from build123d import *

# Parameters (mm, degrees)
F0_R     = 29.980607
F1_DEPTH = 31.75
F2_DEPTH = 17.78
F4_DEPTH = 5.08


with BuildPart() as f1:
    # F0 (on Top) → F1 (new body)
    with BuildSketch(Plane.XY):
        with BuildLine():
            ThreePointArc((8.249651, -24.887905), (54.774032, -39.548346), (83.328802, 0))
            ThreePointArc((83.328802, 0), (54.774032, 39.548346), (8.249651, 24.887905))
            ThreePointArc((8.249651, 24.887905), (2.145128, 13.197838), (0, 0.185486))
            Line((0, 0.185486), (0, 0))
            Line((0, 0), (0, -0.185486))
            ThreePointArc((0, -0.185486), (2.145128, -13.197838), (8.249651, -24.887905))
        make_face()
        with Locations((41.664194, 0)):
            Circle(F0_R, mode=Mode.SUBTRACT)
    extrude(amount=F1_DEPTH)

    # F0 (on Top) → F2 (join)
    with BuildSketch(Plane.XY):
        with BuildLine():
            ThreePointArc((8.249651, -24.887905), (54.774032, -39.548346), (83.328802, 0))
            ThreePointArc((83.328802, 0), (54.774032, 39.548346), (8.249651, 24.887905))
            ThreePointArc((8.249651, 24.887905), (2.145128, 13.197838), (0, 0.185486))
            Line((0, 0.185486), (0, 0))
            Line((0, 0), (0, -0.185486))
            ThreePointArc((0, -0.185486), (2.145128, -13.197838), (8.249651, -24.887905))
        make_face()
        with Locations((41.664194, 0)):
            Circle(F0_R, mode=Mode.SUBTRACT)
        with BuildLine():
            ThreePointArc((0, 0.185486), (2.145128, 13.197838), (8.249651, 24.887905))
            Line((8.249651, 24.887905), (0, 24.887905))
            Line((0, 24.887905), (0, 0.185486))
        make_face()
        with BuildLine():
            Line((0, -24.887905), (8.249651, -24.887905))
            ThreePointArc((8.249651, -24.887905), (2.145128, -13.197838), (0, -0.185486))
            Line((0, -0.185486), (0, -24.887905))
        make_face()
        with BuildLine():
            ThreePointArc((-0.000413, 0), (-0.00031, 0.092743), (0, 0.185486))
            Line((0, 0.185486), (0, 24.887905))
            Line((0, 24.887905), (-76.291874, 24.887905))
            Line((-76.291874, 24.887905), (-76.291874, 0))
            Line((-76.291874, 0), (-0.000413, 0))
        make_face()
        with BuildLine():
            Line((0, -24.887905), (0, -0.185486))
            ThreePointArc((0, -0.185486), (-0.00031, -0.092743), (-0.000413, 0))
            Line((-0.000413, 0), (-76.291874, 0))
            Line((-76.291874, 0), (-76.291874, -24.887905))
            Line((-76.291874, -24.887905), (0, -24.887905))
        make_face()
    extrude(amount=F2_DEPTH)

    # F3 (on Front) → F4 (join, symmetric)
    with BuildSketch(Plane.XZ):
        Polygon((0, 31.850059), (-38.292281, 18.104225), (0, 18.104225), align=None)
    extrude(amount=F4_DEPTH, both=True)


solid = f1.part
Check sheet for the modelled part. Datum: model origin and axes. Units: mm. A direction names the side the tool comes from. Round coordinates to 2 decimals unless told otherwise and drop trailing zeros. Loops run counter-clockwise (first coordinate to the right, second up) from the corner with the lowest first, then second, coordinate; pieces in that order, holes last. Notation, with made-up numbers: (87, -37) -> (114, -37) arc R22 cw to (114, -27) -> close; hole circle Ø10 at (-24.75, 55). An arc over 180 degrees is marked (long way). Put each result on its own line as item: value. Start each with the question number.
1. Gauge pin test, flat ends, axial feed: pin 1 (3 mm diameter, centred on x = -9.5, y = 24.5, fed in from +Z); pin 2 (14 mm diameter, centred on x = -34.5, z = 9, fed in from +Y); pin 3 (15 mm diameter, centred on x = -42, y = 5.5, fed in from +Z). Record the tip position at first contact, or that the pin passes through.
2. Draft check along Z on faces 1 (the face through (13, 10, 31.75)), 2 (the face through (-19, 0, 18.104)), 3 (the face through (-76.292, 0, 9)). Enter one of: +Z half, -Z half, draft (parallel to the pull), parting line (faces both ways), or undercut.
3. Access from +Z, -Z, +X, -X, +Y, -Y to the whole of each face (thin tool, end or side, straight path). Record for faces 4 (the face through (-11, -5.08, 22)), 5 (the face through (-35, -24.888, 9)), 6 (the face through (-11, 5.08, 22)).
4. Section check D-D (z = 24.5). Enter the section's corners in (x, y).
5. Scan lines: probe 1 along Z at (x, y) = (-60.5, 8); probe 2 along Y at (x, z) = (-14.5, 16.5); probe 3 along X at (y, z) = (-8.5, 5). Record each from-to range of solid material in increasing order.
6. Section check A-A (x = 22). Enter the section's corners in (y, z), plus the area to 3 significant figures.
7. Section check C-C (y = 13). Enter the section's corners in (x, z), plus the area to 3 significant figures.
Findings:
1. pin 1: stops at z = 17.78
1. pin 2: stops at y = 24.89
1. pin 3: stops at z = 19.46
2. face 1: +Z half
2. face 2: undercut
2. face 3: draft
3. face 4: +Z, -X, -Y
3. face 5: +Z, -Z, -X, -Y
3. face 6: +Z, -X, +Y
4. outline: (-20.48, -5.08) -> (0, -5.08) -> (0, -0.19) arc R41.66 ccw to (8.25, -24.89) arc R41.66 ccw (long way) to (8.25, 24.89) arc R41.66 ccw to (0, 0.19) -> (0, 5.08) -> (-20.48, 5.08) -> close; hole circle Ø59.96 at (41.66, 0)
5. probe 1: z = 0 to 17.78
5. probe 2: y = -24.89 to 24.89
5. probe 3: x = -76.29 to 12.91, 70.41 to 82.45
6. outline: (-36.73, 0) -> (-22.63, 0) -> (-22.63, 31.75) -> (-36.73, 31.75) -> close; (22.63, 0) -> (36.73, 0) -> (36.73, 31.75) -> (22.63, 31.75) -> close
6. area: 895 mm^2
7. outline: (-76.29, 0) -> (14.65, 0) -> (14.65, 31.75) -> (2.08, 31.75) -> (2.08, 17.78) -> (-76.29, 17.78) -> close; (68.68, 0) -> (81.25, 0) -> (81.25, 31.75) -> (68.68, 31.75) -> close
7. area: 2,190 mm^2
